Source: CAD feature listing. Evaluate the final solid. Frame: model axes, mm. A direction names the side the tool comes from. Round coordinates to 2 decimals unless told otherwise and drop trailing zeros. Loops run counter-clockwise (first coordinate to the right, second up) from the corner with the lowest first, then second, coordinate; pieces in that order, holes last.
(1) Section D-D, the plane z = -15.5. Return the cut outline in (x, y).
(2) Set-up query: faces 1 (the cylindrical face through (-19.27, 16.09, -40.68)), 2 (the cylindrical face through (9.42, 33.49, -8.06)), 3 (the flat face through (-11, 35, -12)), 4 (the cylindrical face through (7.757, -4.465, -4.84)), 5 (the flat face through (16, 15, -13.091)). Return all of +Z, -Z, +X, -X, +Y, -Y with unobstructed straight access to the full face (end or side cutting, diameter ignored); none if empty.
(3) First-contact query: pin 1 Ø10 at (y, z) = (12.5, -28.5) entering from -X; pin 2 Ø0.6 at (x, y) = (-11, 38.5) entering from -Z; pin 3 Ø1.5 at (y, z) = (35.5, -8) entering from -X; pin 4 Ø5 at (y, z) = (3, -12) entering from +X. Flat tips, straight axial feed; report the tip coordinate or a pass-through.
(4) Material intervals for probe 1 along Y at (x, z) = (4.5, -19); probe 2 along Y at (x, z) = (-4, -7); probe 3 along Z at (x, y) = (4, 34.5), sorted ascending.
(5) Section B-B, the plane x = 14. Return the cut outline in (y, z), plus the area to 3 significant figures.
(6) Section A-A, the plane z = -8.7. Return the cut outline in (x, y), plus the area to 3 significant figures.
(7) Mould query, pull axis X, two halves, no side actions, for faces 6 (the cylindrical face through (-20.06, 15.91, -16.1)), 7 (the flat face through (-15.01, 31.8, -35.81)), 8 (the flat face through (11, 35, -12)). Classes: pulls with the +X half, pulls with the -X half, needs draft (parallel to the pull), parting line crosses it, or undercut.
(8) Section C-C, the plane y = 11.5. Return the cut outline in (x, z), plus the area to 3 significant figures.
```python
from build123d import *

# Parameters (mm, degrees)
BOSS_EXTRUDE1_DEPTH     = 32.5
SKETCH4_R               = 1.05
BOSS_EXTRUDE2_DEPTH     = 2
SKETCH7_R               = 2.495
WIRE_SPACING2_DEPTH     = 3
SKETCH8_W               = 30.122
SKETCH8_H               = 37.7
SKETCH8_R               = 2.495
BOSS_EXTRUDE6_DEPTH     = 2
SKETCH5_R               = 1.05
BOSS_EXTRUDE3_DEPTH     = 2
SKETCH9_R               = 2.495
WIRE_SPACING1_DEPTH     = 3
SKETCH10_W              = 30.122
SKETCH10_H              = 37.7
SKETCH10_R              = 2.495
BOSS_EXTRUDE8_DEPTH     = 2
SKETCH11_R              = 12.5
CUT_EXTRUDE1_DEPTH      = 47.5
SKETCH18_W              = 10
SKETCH18_H              = 10
CUT_EXTRUDE4_DEPTH      = 47.5
BOSS_EXTRUDE10_DEPTH    = 2.5
BOSS_EXTRUDE11_DEPTH    = 2.5
BOSS_EXTRUDE12_DEPTH    = 43.7
CUT_EXTRUDE5_DEPTH      = 21.061
CUT_EXTRUDE5_DEPTH_BACK = 21.061
CUT_EXTRUDE7_DEPTH      = 8.5
CUT_EXTRUDE8_DEPTH      = 47.5


with BuildPart() as part:
    # Sketch2 → Boss-Extrude1 (new body)
    with BuildSketch(Plane(origin=(0, 0, 0), x_dir=(1, 0, 0), z_dir=(0, 1, 0))):
        Polygon((15.061, 0), (15.061, 37.7), (12.561, 37.7), (12.561, 2.5), (-12.561, 2.5), (-12.561, 37.7), (-15.061, 37.7), (-15.061, 0), align=None)
    extrude(amount=BOSS_EXTRUDE1_DEPTH)

    # Sketch4 → Boss-Extrude2 (add)
    with BuildSketch(Plane.XZ):
        Polygon((-15.061, 0), (-15.061, -7.443777264), (-15.061, -37.7), (-12.561, -37.7), (-12.561, -7.5), (12.561, -7.5), (12.561, -37.7), (15.061, -37.7), (15.061, -7.443777264), (15.061, 0), align=None)
        with Locations((-10.2499, -4.95)):
            Circle(SKETCH4_R, mode=Mode.SUBTRACT)
        with Locations((10.2499, -4.95)):
            Circle(SKETCH4_R, mode=Mode.SUBTRACT)
    extrude(amount=BOSS_EXTRUDE2_DEPTH)

    # Sketch7 → Wire spacing2 (add)
    with BuildSketch(Plane.XZ.offset(2)):
        Polygon((-15.061, 0), (-15.061, -37.7), (-12.561, -37.7), (-12.561, -7.5), (12.561, -7.5), (12.561, -37.7), (15.061, -37.7), (15.061, 0), align=None)
        with Locations((-10.2499, -4.95)):
            Circle(SKETCH7_R, mode=Mode.SUBTRACT)
        with Locations((10.2499, -4.95)):
            Circle(SKETCH7_R, mode=Mode.SUBTRACT)
    extrude(amount=WIRE_SPACING2_DEPTH)

    # Sketch8 → Boss-Extrude6 (add)
    with BuildSketch(Plane.XZ.offset(5)):
        with Locations((0, -18.85)):
            Rectangle(SKETCH8_W, SKETCH8_H)
        with Locations((-10.2499, -4.95)):
            Circle(SKETCH8_R, mode=Mode.SUBTRACT)
        with Locations((10.2499, -4.95)):
            Circle(SKETCH8_R, mode=Mode.SUBTRACT)
    extrude(amount=BOSS_EXTRUDE6_DEPTH)

    # Sketch5 → Boss-Extrude3 (add)
    with BuildSketch(Plane(origin=(0, 32.5, 0), x_dir=(1, 0, 0), z_dir=(0, 1, 0))):
        Polygon((-7.5, 10), (-7.5, 2.5), (7.5, 2.5), (7.5, 10), (10.2499, 12), (12.561, 12), (12.561, 37.7), (15.061, 37.7), (15.061, 0), (-15.061, 0), (-15.061, 37.7), (-12.561, 37.7), (-12.561, 12), (-10.2499, 12), align=None)
        with Locations((-10.2499, 8.7)):
            Circle(SKETCH5_R, mode=Mode.SUBTRACT)
        with Locations((10.2499, 8.7)):
            Circle(SKETCH5_R, mode=Mode.SUBTRACT)
    extrude(amount=BOSS_EXTRUDE3_DEPTH)

    # Sketch9 → Wire spacing1 (add)
    with BuildSketch(Plane(origin=(0, 34.5, 0), x_dir=(1, 0, 0), z_dir=(0, 1, 0))):
        Polygon((-15.061, 0), (-15.061, 37.7), (-12.561, 37.7), (-12.561, 12), (-10.2499, 12), (-7.5, 10), (-7.5, 2.5), (7.5, 2.5), (7.5, 10), (10.2499, 12), (12.561, 12), (12.561, 37.7), (15.061, 37.7), (15.061, 0), align=None)
        with Locations((-10.2499, 8.7)):
            Circle(SKETCH9_R, mode=Mode.SUBTRACT)
        with Locations((10.2499, 8.7)):
            Circle(SKETCH9_R, mode=Mode.SUBTRACT)
    extrude(amount=WIRE_SPACING1_DEPTH)

    # Sketch10 → Boss-Extrude8 (add)
    with BuildSketch(Plane(origin=(0, 37.5, 0), x_dir=(1, 0, 0), z_dir=(0, 1, 0))):
        with Locations((0, 18.85)):
            Rectangle(SKETCH10_W, SKETCH10_H)
        with Locations((-10.2499, 8.7)):
            Circle(SKETCH10_R, mode=Mode.SUBTRACT)
        with Locations((10.2499, 8.7)):
            Circle(SKETCH10_R, mode=Mode.SUBTRACT)
    extrude(amount=BOSS_EXTRUDE8_DEPTH)

    # Sketch11 → Cut-Extrude1 (cut, through all)
    with BuildSketch(Plane(origin=(0, 39.5, 0), x_dir=(1, 0, 0), z_dir=(0, 1, 0))):
        with Locations((0, 37.7)):
            Circle(SKETCH11_R)
    extrude(amount=-CUT_EXTRUDE1_DEPTH, mode=Mode.SUBTRACT)

    # Sketch18 → Cut-Extrude4 (cut, through all)
    with BuildSketch(Plane(origin=(0, 39.5, 0), x_dir=(1, 0, 0), z_dir=(0, 1, 0))):
        with Locations((-10.061, 32.7)):
            Rectangle(SKETCH18_W, SKETCH18_H)
        with Locations((10.061, 32.7)):
            Rectangle(SKETCH18_W, SKETCH18_H)
    extrude(amount=-CUT_EXTRUDE4_DEPTH, mode=Mode.SUBTRACT)

    # Sketch19 → Boss-Extrude10 (add)
    with BuildSketch(Plane.ZY.offset(15.061)):
        Polygon((-27.7, 37.5), (-43.7, 26.25), (-43.7, 6.25), (-27.7, -5), align=None)
    extrude(amount=-BOSS_EXTRUDE10_DEPTH)

    # Sketch20 → Boss-Extrude11 (add)
    with BuildSketch(Plane(origin=(15.061, 0, 0), x_dir=(0, 0, -1), z_dir=(1, 0, 0))):
        Polygon((27.7, 37.5), (43.7, 26.25), (43.7, 6.25), (27.7, -5), align=None)
    extrude(amount=-BOSS_EXTRUDE11_DEPTH)

    # Sketch21 → Boss-Extrude12 (add)
    with BuildSketch(Plane.XY):
        with BuildLine():
            Line((15.061, 39.5), (15.061, -7))
            ThreePointArc((15.061, -7), (20.061, 16.25), (15.061, 39.5))
        make_face()
        with BuildLine():
            Line((-15.061, 39.5), (-15.061, -7))
            ThreePointArc((-15.061, -7), (-20.061, 16.25), (-15.061, 39.5))
        make_face()
    extrude(amount=-BOSS_EXTRUDE12_DEPTH)

    # Sketch22 → Cut-Extrude5 (cut, two sides)
    with BuildSketch(Plane(origin=(0, 0, 0), x_dir=(0, 0, -1), z_dir=(1, 0, 0))) as cut_extrude5_sk:
        Polygon((27.7, 37.5), (27.7, 39.5), (50.372745126, 39.5), (50.372745126, -11.616849197), (27.7, -11.616849197), (27.7, -5), (43.7, 6.25), (43.7, 26.25), align=None)
    extrude(amount=CUT_EXTRUDE5_DEPTH, mode=Mode.SUBTRACT)
    extrude(cut_extrude5_sk.sketch, amount=-CUT_EXTRUDE5_DEPTH_BACK, mode=Mode.SUBTRACT)

    # Sketch23 → Cut-Extrude7 (cut, through all)
    with BuildSketch(Plane.ZY.offset(-12.561)):
        Polygon((-27.7, 37.5), (-13.091239011, 21.881848889), (-13.091239011, 8.292742538), (-27.7, -5), (-48.045036631, -3.33430033), (-49.353078953, 36.560990509), align=None)
    extrude(amount=-CUT_EXTRUDE7_DEPTH, mode=Mode.SUBTRACT)

    # Sketch24 → Cut-Extrude8 (cut, through all)
    with BuildSketch(Plane.XZ.offset(7)):
        with BuildLine():
            Line((-19.53, -76.468982583), (19.53, -77.324698996))
            Line((19.53, -77.324698996), (19.53, -37.5))
            ThreePointArc((19.53, -37.5), (0, -57.03), (-19.53, -37.5))
            Line((-19.53, -37.5), (-36.23071583, -37.5))
            Line((-36.23071583, -37.5), (-36.23071583, -76.468982583))
            Line((-36.23071583, -76.468982583), (-19.53, -76.468982583))
        make_face()
    extrude(amount=-CUT_EXTRUDE8_DEPTH, mode=Mode.SUBTRACT)


solid = part.part
```
Output values:
1. outline: (-15.06, -7) - (15.06, -7) arc R56.56 ccw to (19.14, 6.1) - (12.56, 6.1) - (12.56, -5) - (-12.56, -5) - (-12.56, 37.5) - (12.56, 37.5) - (12.56, 24.46) - (19.46, 24.46) arc R56.56 ccw to (15.06, 39.5) - (-15.06, 39.5) arc R56.56 ccw to start
2. face 1: -Z, -X, +Y, -Y
2. face 2: +Y
2. face 3: -Z
2. face 4: -Y
2. face 5: -Z, +X
3. pin 1: stops at x = -20.06
3. pin 2: stops at z = -27.7
3. pin 3: stops at x = -16.95
3. pin 4: stops at x = 19.03
4. probe 1: y = -7 to -5, 37.5 to 39.5
4. probe 2: y = -7 to 0, 37.5 to 39.5
4. probe 3: z = -2.5 to 0
5. outline: (-7, -27.7) - (-5, -27.7) - (8.29, -13.09) - (21.88, -13.09) - (37.5, -27.7) - (39.5, -27.7) - (39.5, 0) - (-7, 0) - close
5. area: 878 mm2
6. outline: (-15.06, -7) - (15.06, -7) arc R56.56 ccw to (15.06, 39.5) - (12.74, 39.5) - (12.74, 34.5) - (11.3, 34.5) - (11.3, 32.5) - (12.56, 32.5) - (12.56, -5) - (-12.56, -5) - (-12.56, 32.5) - (-11.3, 32.5) - (-11.3, 34.5) - (-12.74, 34.5) - (-12.74, 39.5) - (-15.06, 39.5) arc R56.56 ccw to start; (-9.2, 32.5) - (-7.5, 32.5) - (-7.5, 37.5) - (7.5, 37.5) - (7.5, 32.5) - (9.2, 32.5) - (9.2, 34.5) - (7.75, 34.5) - (7.75, 39.5) - (-7.75, 39.5) - (-7.75, 34.5) - (-9.2, 34.5) - close
6. area: 638 mm2
7. face 6: pulls with the -X half
7. face 7: needs draft
7. face 8: undercut
8. outline: (-19.86, -37.5) - (-19.53, -37.5) arc R19.53 ccw to (-18.52, -43.7) - (-12.56, -43.7) - (-12.56, -2.5) - (12.56, -2.5) - (12.56, -13.09) - (19.86, -13.09) - (19.86, 0) - (-19.86, 0) - close
8. area: 473 mm2
